Job drawing, mm, ordinate dimensions from the low corner. One solid piece. A direction names the side the tool comes from. Coordinates: 2 decimals unless noted, no trailing zeros. Write each loop counter-clockwise with the first axis right and the second up, starting at its lowest first coordinate (ties: lowest second). Pieces come first, ordered by that corner, then holes.
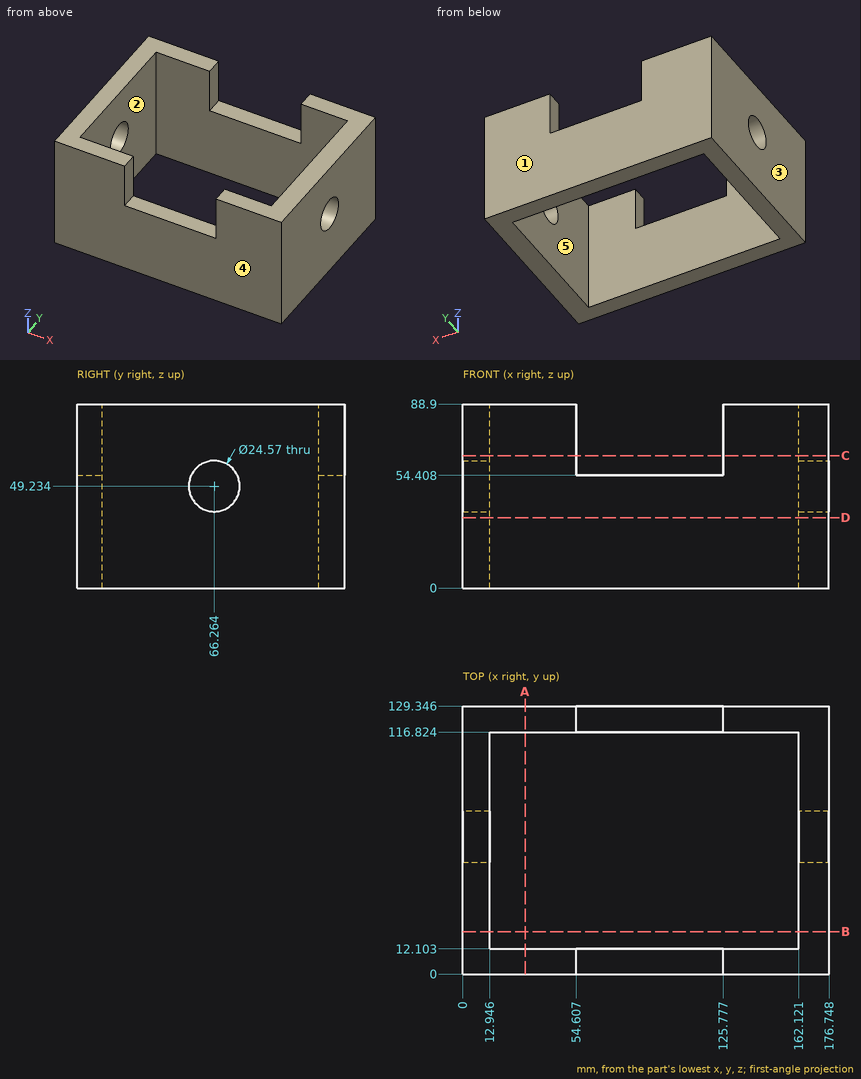
1. Saw through at B-B on y = 20.5. List the corners of the cut face in (x, z) (1 decimal), plus the area to 3 significant figures.
Computed values:
outline: (0, 0) - (12.9, 0) - (12.9, 88.9) - (0, 88.9) - close; (162.1, 0) - (176.7, 0) - (176.7, 88.9) - (162.1, 88.9) - close
area: 2,450 mm2
2. Saw through at C-C on z = 64. List the corners of the cut face in (x, y) (1 decimal).
Computed values:
outline: (0, 0) - (54.6, 0) - (54.6, 12.1) - (12.9, 12.1) - (12.9, 116.8) - (54.6, 116.8) - (54.6, 129.3) - (0, 129.3) - close; (125.8, 0) - (176.7, 0) - (176.7, 129.3) - (125.8, 129.3) - (125.8, 116.8) - (162.1, 116.8) - (162.1, 12.1) - (125.8, 12.1) - close
3. Mould opens along Y. For the marked faces 3, 4 and 5 say: +Y half, -Y half, draft (parallel to the pull), parting line (faces both ways), or undercut.
Computed values:
face 3: draft
face 4: -Y half
face 5: undercut
4. 3-axis set-ups, long thin cutter, end or side, ignore diameter. For the marked faces 1 and 2: which of +Z, -Z, +X, -X, +Y, -Y reach the whole face in a straight line?
Computed values:
face 1: +Z, -Z, +X, -X, +Y
face 2: +Z, -Z
5. Flat gauge pin, fed straight in: pin 1 (14 mm diameter, centred on x = 94, y = 125.5, fed in from +Z). Where does the tip first touch, or does it go through?
Computed values:
pin 1: stops at z = 54.41
6. Saw through at A-A on x = 30. List the corners of the cut face in (y, z) (1 decimal), plus the area to 3 significant figures.
Computed values:
outline: (0, 0) - (12.1, 0) - (12.1, 88.9) - (0, 88.9) - close; (116.8, 0) - (129.3, 0) - (129.3, 88.9) - (116.8, 88.9) - close
area: 2,190 mm2
7. Saw through at D-D on z = 34. List the corners of the cut face in (x, y) (1 decimal).
Computed values:
outline: (0, 0) - (176.7, 0) - (176.7, 129.3) - (0, 129.3) - close; hole (12.9, 12.1) - (162.1, 12.1) - (162.1, 116.8) - (12.9, 116.8) - close
8. Probe line 1 along X through (y, z) = (61, 76.5) (1 decimal); line 2 along Y through (x, z) = (46.5, 20.5) (1 decimal); line 3 along Z through (x, y) = (87.5, 117). List the from-to ranges inside material, lowest first.
Computed values:
line 1: x = 0 to 12.9, 162.1 to 176.7
line 2: y = 0 to 12.1, 116.8 to 129.3
line 3: z = 0 to 54.41
